The model under review builds one solid part; all positions refer to its coordinate system, in mm. A direction names the side the tool comes from. Round coordinates to 2 decimals unless told otherwise and drop trailing zeros. Write each loop counter-clockwise with the first axis right and the second up, starting at its lowest first coordinate (ties: lowest second). Pieces come first, ordered by that corner, then holes. Notation, with made-up numbers: (39.5, 63.5) - (44.5, 63.5) arc R17 cw to (44.5, 87.5) - close; hole circle Ø5 at (66, 85). An arc over 180 degrees is marked (long way). Use one line per item in the form item = value.
from build123d import *

# Parameters (mm, degrees)
F1_DEPTH = 6.35
F2_R     = 2.413
F3_DEPTH = 6.351


with BuildPart() as f1:
    # F0 (on Top) → F1 (new body)
    with BuildSketch(Plane.XY):
        with BuildLine():
            Line((-6.35, 6.985), (-6.35, 0))
            Line((-6.35, 0), (-6.35, -6.985))
            Line((-6.35, -6.985), (0, -6.985))
            Line((0, -6.985), (0, -10.668))
            Line((0, -10.668), (25.4, -10.668))
            ThreePointArc((25.4, -10.668), (27.579726, -10.656309), (29.759202, -10.621236))
            Line((29.759202, -10.621236), (169.70847, -7.618246))
            ThreePointArc((169.70847, -7.618246), (174.990642, -5.330045), (177.165, 0))
            ThreePointArc((177.165, 0), (174.990642, 5.330045), (169.70847, 7.618246))
            Line((169.70847, 7.618246), (29.759202, 10.621236))
            ThreePointArc((29.759202, 10.621236), (27.579726, 10.656309), (25.4, 10.668))
            Line((25.4, 10.668), (0, 10.668))
            Line((0, 10.668), (0, 6.985))
            Line((0, 6.985), (-6.35, 6.985))
        make_face()
    extrude(amount=F1_DEPTH)

    # F2 (on face) → F3 (cut, through all)
    with BuildSketch(Plane.XY.offset(6.35)):
        with Locations((169.545, 0)):
            Circle(F2_R)
    extrude(amount=-F3_DEPTH, mode=Mode.SUBTRACT)


solid = f1.part
(1) Insertion check: P1, Ø1.8, axis at y = -8.5, z = 4, coming from the -X side; P2, Ø1.9, axis at x = -2, z = 3, coming from the -Y side (3 decimals). Each pin has a flat end and moves straight along its axis. Give the tip position at first contact, or say it passes through.
Geometry results:
P1 = 0
P2 = -6.985
(2) The part is to be moulded in two halves that separate along Y. For faces 1 (the cylindrical face through (171.85, 0.72, 3.22)), 2 (the cylindrical face through (27.549, -10.657, 3.131)), 3 (the flat face through (-3, 6.985, 3)), say which applies: +Y half, -Y half, draft (parallel to the pull), parting line (faces both ways), or undercut.
Geometry results:
face_1 = undercut
face_2 = -Y half
face_3 = +Y half
(3) Add section A-A on z = 1.75. Write out the cut boundary in (x, y) (3 decimals).
Geometry results:
outline = (-6.35, -6.985) - (0, -6.985) - (0, -10.668) - (25.4, -10.668) arc R203.194 ccw to (29.759, -10.621) - (169.708, -7.618) arc R7.62 ccw to (169.708, 7.618) - (29.759, 10.621) arc R203.194 ccw to (25.4, 10.668) - (0, 10.668) - (0, 6.985) - (-6.35, 6.985) - close; hole circle Ø4.826 at (169.545, 0)
(4) Machinability: for faces 4 (the flat face through (0, 9, 3)), 5 (the flat face through (0, -9, 3)), 6 (the flat face through (13, -10.668, 3)), which of the approach directions +Z, -Z, +X, -X, +Y, -Y give a long, thin tool a straight path to every point of the face, cutting with its end or side? Answer none if there is none.
Geometry results:
face_4 = +Z, -Z, -X, +Y
face_5 = +Z, -Z, -X, -Y
face_6 = +Z, -Z, +X, -X, -Y
(5) Add section B-B on x = 68. Write out the cut boundary in (y, z), then the cut area to 3 significant figures.
Geometry results:
outline = (-9.8, 0) - (9.8, 0) - (9.8, 6.35) - (-9.8, 6.35) - close
area = 124 mm2
(6) Add section C-C on x = 103.5. Write out the cut boundary in (y, z).
Geometry results:
outline = (-9.04, 0) - (9.04, 0) - (9.04, 6.35) - (-9.04, 6.35) - close
(7) To check wall thickness, follow L1, parallel to Y at x = 26.5, z = 3.5; L2, parallel to Y at x = 168, z = 5.75; L3, parallel to X at y = -1.5, z = 2.25. State the ranges of each line that lie inside material, in increasing order.
Geometry results:
L1 = -10.67 to 10.67
L2 = -7.65 to -1.85, 1.85 to 7.65
L3 = -6.35 to 167.65, 171.44 to 177.02
